```python
from build123d import *

# Parameters (mm, degrees)
P_IDAT_VYSUNUT_M1_DEPTH  = 79.2
SKICA2_W                 = 5.1
SKICA2_H                 = 13
ODEBRAT_VYSUNUT_M1_DEPTH = 10
ODEBRAT_VYSUNUT_M2_DEPTH = 6.65


with BuildPart() as part:
    # Skica1 → Přidat vysunutím1 (new body)
    with BuildSketch(Plane.XY):
        with BuildLine():
            Line((0, 24.2), (33.2, 24.2))
            ThreePointArc((33.2, 24.2), (45.3, 12.1), (33.2, 0))
            Line((33.2, 0), (0, 0))
            ThreePointArc((0, 0), (-12.1, 12.1), (0, 24.2))
        make_face()
    extrude(amount=P_IDAT_VYSUNUT_M1_DEPTH)

    # Skica2 → Odebrat vysunutím1 (cut)
    with BuildSketch(Plane(origin=(0, 0, 0), x_dir=(-1, 0, 0), z_dir=(0, 0, -1))):
        with Locations((5.15, 12.1)):
            Rectangle(SKICA2_W, SKICA2_H)
    extrude(amount=-ODEBRAT_VYSUNUT_M1_DEPTH, mode=Mode.SUBTRACT)

    # Skica3 → Odebrat vysunutím2 (cut)
    with BuildSketch(Plane.XY.offset(79.2)):
        with BuildLine():
            Line((-7.1, 9.2), (-7.1, 15))
            ThreePointArc((-7.1, 15), (-5.8, 16.3), (-4.5, 15))
            Line((-4.5, 15), (-4.5, 9.2))
            ThreePointArc((-4.5, 9.2), (-5.8, 7.9), (-7.1, 9.2))
        make_face()
    extrude(amount=-ODEBRAT_VYSUNUT_M2_DEPTH, mode=Mode.SUBTRACT)


solid = part.part
```
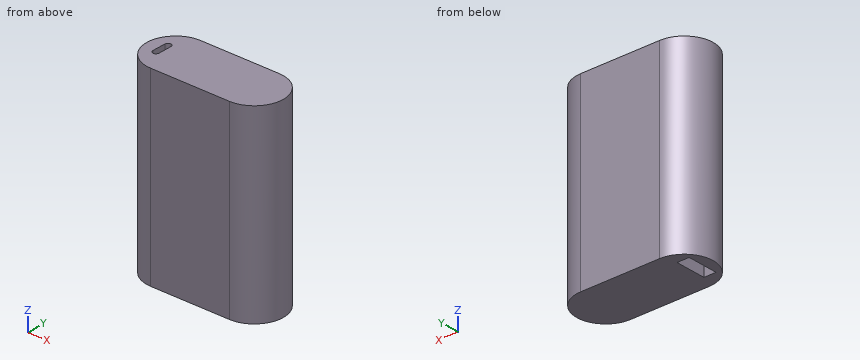
Could you check a few things on this model? Use its own coordinates, in mm. Round coordinates to 2 decimals unless told otherwise and drop trailing zeros. Order: outer loops, then holes, each group sorted by start corner. A loop starts at its lowest first (then second) coordinate and runs counter-clockwise, first axis right, second up. Notation, with made-up numbers: (83.5, 26) -> (100.5, 26) arc R21 ccw to (100.5, 41) -> close; hole circle Ø5 at (35.5, 23). An arc over 180 degrees is marked (long way). One line per question, with ' | ' between items.
Q1. If we section it at C-C on z = 71: Write out the boundary of the cut face in (x, y).
Computed values:
outline: (0, 0) -> (33.2, 0) arc R12.1 ccw to (33.2, 24.2) -> (0, 24.2) arc R12.1 ccw to start
Q2. If we section it at A-A on x = -5.8: Write out the boundary of the cut face in (y, z).
Computed values:
outline: (1.48, 0) -> (5.6, 0) -> (5.6, 10) -> (18.6, 10) -> (18.6, 0) -> (22.72, 0) -> (22.72, 79.2) -> (16.3, 79.2) -> (16.3, 72.55) -> (7.9, 72.55) -> (7.9, 79.2) -> (1.48, 79.2) -> close
Q3. If we section it at D-D on x = 42.5: Write out the boundary of the cut face in (y, z), plus the area to 3 significant figures.
Computed values:
outline: (4.36, 0) -> (19.84, 0) -> (19.84, 79.2) -> (4.36, 79.2) -> close | area: 1,230 mm²
Q4. If I drill on line 1 (Y direction, x = -4.5, z = 9); line 2 (X direction, y = 12, z = 52.5); line 3 (Y direction, x = 38, z = 58), over which ranges is the centre line in solid material (lowest first)? Write a range as from..to.
Computed values:
line 1: 0.87..5.6, 18.6..23.33 | line 2: -12.1..45.3 | line 3: 0.99..23.21
Q5. If we section it at B-B on y = 7: Write out the boundary of the cut face in (x, z).
Computed values:
outline: (-10.97, 0) -> (-7.7, 0) -> (-7.7, 10) -> (-2.6, 10) -> (-2.6, 0) -> (44.17, 0) -> (44.17, 79.2) -> (-10.97, 79.2) -> close
Q6. I'm going to push flat-ended pins straight in: pin 1 (4 mm diameter, centred on x = -4, z = 5, fed in from +Y); pin 2 (1.3 mm diameter, centred on x = -5.5, y = 13.5, fed in from +Z); pin 3 (1.5 mm diameter, centred on x = -6, z = 4.5, fed in from -Y). Where does each tip first touch, or does it pass through?
Computed values:
pin 1: y = 24.03 | pin 2: z = 72.55 | pin 3: y = 1.2
